Could you check a few things on this model? Use its own coordinates, in mm. Face numbers are marked on the shaded views. Round coordinates to 2 decimals unless told otherwise and drop trailing zeros. Order: outer loops, then holes, each group sorted by start corner. A loop starts at its lowest first (then second) coordinate and runs counter-clockwise, first axis right, second up. Notation, with made-up numbers: (69, 64.5) -> (111, 64.5) arc R15 ccw to (111, 69.5) -> close; hole circle Ø7 at (4, 51.5). An arc over 180 degrees is marked (long way). One line per question, with ' | ' between items.
```python
from build123d import *

# Parameters (mm, degrees)
SKETCH_7_R          = 40
CUT_EXTRUDE_1_DEPTH = 73.864118401
SKETCH_8_R          = 1.5
CUT_EXTRUDE_2_DEPTH = 10


with BuildPart() as part:
    # 草图5 → 旋转2 (revolve)
    with BuildSketch(Plane.XY, mode=Mode.PRIVATE) as revolve_2_sk:
        with BuildLine():
            Line((-46.752169664, 16.788080184), (2.247830336, 16.788080184))
            Line((2.247830336, 16.788080184), (2.247830336, 8.488080184))
            Line((2.247830336, 8.488080184), (-46.752169664, 8.488080184))
            Line((-46.752169664, 8.488080184), (-46.752169664, 11.319510864))
            ThreePointArc((-46.752169664, 11.319510864), (-46.381680312, 11.906305273), (-46.252169664, 12.588080184))
            ThreePointArc((-46.252169664, 12.588080184), (-46.381680312, 13.269855096), (-46.752169664, 13.856649505))
            Line((-46.752169664, 13.856649505), (-46.752169664, 16.788080184))
        make_face()
    revolve(revolve_2_sk.sketch.rotate(Axis((2.247830336, 16.788080184, 0), (0, -1, 0)), 270), axis=Axis((2.247830336, 16.788080184, 0), (0, -1, 0)))

    # 草图7 → 切除-拉伸1 (cut, through all)
    with BuildSketch(Plane(origin=(0, 0, 0), x_dir=(1, 0, 0), z_dir=(0, 1, 0))):
        with Locations(Location((2.247830336, 0, 0), (0, 0, 90))):
            Circle(SKETCH_7_R)
    extrude(amount=CUT_EXTRUDE_1_DEPTH, mode=Mode.SUBTRACT)

    # 草图8 → 切除-拉伸2 (cut)
    with BuildSketch(Plane(origin=(0, 16.788080184, 0), x_dir=(1, 0, 0), z_dir=(0, 1, 0))):
        with Locations(Location((2.247830336, 44.5, 0), (0, 0, 270))):
            Circle(SKETCH_8_R)
        with Locations(Location((46.747830336, 0, 0), (0, 0, 270))):
            Circle(SKETCH_8_R)
        with Locations(Location((2.247830336, -44.5, 0), (0, 0, 270))):
            Circle(SKETCH_8_R)
        with Locations(Location((-42.252169664, 0, 0), (0, 0, 270))):
            Circle(SKETCH_8_R)
    extrude(amount=-CUT_EXTRUDE_2_DEPTH, mode=Mode.SUBTRACT)


solid = part.part
```
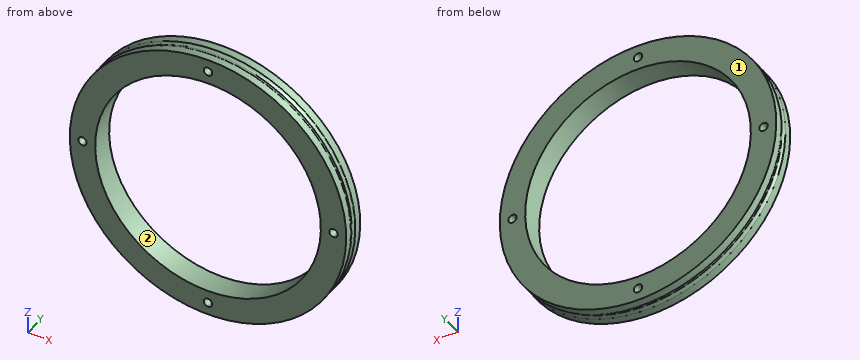
1. I'm going to push flat-ended pins straight in: pin 1 (1.5 mm diameter, centred on x = -25, y = 10.5, fed in from -Z); pin 2 (4 mm diameter, centred on y = 11.5, z = 31, fed in from +X). Where does each tip first touch, or does it pass through?
From the geometry:
pin 1: stops at z = -41.22 | pin 2: stops at x = 41.74
2. If we mould it in two halves opening along Z, with no side actions, what happens to the marked faces 1 and 2? For each: pulls with the +Z half, pulls with the -Z half, needs draft (parallel to the pull), parting line crosses it, or undercut.
From the geometry:
face 1: needs draft | face 2: undercut
3. I need wall thicknesses on probe 1 along X at (y, z) = (11, 0); probe 2 along Z at (x, y) = (3, 11.25); probe 3 along X at (y, z) = (12.25, 0). Which ranges of each line are inside material? Lowest first, please.
From the geometry:
probe 1: x = -46.75 to -43.75, -40.75 to -37.75, 42.25 to 45.25, 48.25 to 51.25 | probe 2: z = -48.99 to -45.8, -43.2 to -39.99, 39.99 to 43.2, 45.8 to 48.99 | probe 3: x = -46.28 to -43.75, -40.75 to -37.75, 42.25 to 45.25, 48.25 to 50.78
4. I want a section at A-A on y = 15.25. List the corners of the cut face in (x, z) for me, and give its area (3 significant figures).
From the geometry:
outline: circle Ø98 at (2.25, 0); hole circle Ø3 at (-42.25, 0); hole circle Ø80 at (2.25, 0); hole circle Ø3 at (2.25, -44.5); hole circle Ø3 at (2.25, 44.5); hole circle Ø3 at (46.75, 0) | area: 2,490 mm²
